The listing builds one solid part. Answer for the finished solid, in the listing's coordinates (mm). A direction names the side the tool comes from. Give positions to 0.01 mm unless a question says otherwise; leave off trailing zeros. Write each loop counter-clockwise with the first axis right and the second up, starting at its lowest first coordinate (ties: lowest second). Pieces come first, ordered by that corner, then holes. Notation, with made-up numbers: M 36,25 L 51,25 A26 ccw 51,40 Z; hole C -0.75,56 d4. An arc over 180 degrees is marked long. Return JSON: item names as keys, results as strings.
from build123d import *

# Parameters (mm, degrees)
F0_W = 99.274278
F0_H = 45.48195
F2_R = 20.32
F3_T = -2.54


with BuildPart() as f1:
    # F0 (on Right) → F1 (revolve)
    with BuildSketch(Plane.YZ):
        with Locations((49.637139, 22.740975)):
            Rectangle(F0_W, F0_H)
    revolve(axis=Axis((0, 49.637139, 0), (0, 1, 0)))

    # F2
    f2_edges = [f1.edges().sort_by_distance(p)[0] for p in [
        (0, 0, -45.48195),
    ]]
    fillet(f2_edges, radius=F2_R)

    # F3
    f3_openings = [f1.faces().sort_by_distance(p)[0] for p in [
        (0, 99.274278, 0),
    ]]
    offset(amount=F3_T, openings=f3_openings)


solid = f1.part
Item 1: A cutting plane is placed at C-C, the plane y = 79. Write down the section's boundary in (x, z), plus the area to 3 significant figures.
Geometry results:
{"outline": "C 0,0 d90.96; hole C 0,0 d85.88", "area": "706 mm2"}
Item 2: A cutting plane is placed at A-A, the plane z = 0. Write down the section's boundary in (x, y), plus the area to 3 significant figures.
Geometry results:
{"outline": "M -45.48,20.32 A20.32 ccw -25.16,0 L 25.16,0 A20.32 ccw 45.48,20.32 L 45.48,99.27 L 42.94,99.27 L 42.94,20.32 A17.78 cw 25.16,2.54 L -25.16,2.54 A17.78 cw -42.94,20.32 L -42.94,99.27 L -45.48,99.27 Z", "area": "681 mm2"}
Item 3: Find the intervals of material crossed by line 1 (X direction, y = 78.5, z = 0); line 2 (Y direction, x = -1, z = 25.5); line 3 (Z direction, x = -17, y = 66), in increasing order.
Geometry results:
{"line 1": "x = -45.48 to -42.94, 42.94 to 45.48", "line 2": "y = 0 to 2.54", "line 3": "z = -42.19 to -39.43, 39.43 to 42.19"}
Item 4: Given pin 1 Ø8 at (x, z) = (27, 19) entering from +Y; pin 2 Ø4 at (x, y) = (-27.5, 43.5) entering from -Z; pin 3 Ø4 at (y, z) = (21.5, -7) entering from -X, each flat-ended and moving along its own axis, determine where each tip first touches the part or whether it passes through.
Geometry results:
{"pin 1": "stops at y = 7.07", "pin 2": "stops at z = -37.66", "pin 3": "stops at x = -45.21"}
Item 5: Which of the six approach directions +Z, -Z, +X, -X, +Y, -Y give full straight-line access (tool end or side, diameter ignored) to faces 4 (the cylindrical face through (12.9, 60.35, 40.96)), 5 (the flat face through (0, 0, 0))?
Geometry results:
{"face 4": "+Y", "face 5": "+Z, -Z, +X, -X, -Y"}
Item 6: Determine the mould class of faces 1 (the flat face through (27.2, 99.274, -33.5)), 2 (the cylindrical face through (13.662, 60.35, 43.382)), 3 (the flat face through (0, 2.54, 0)) for opening direction Z: +Z half, -Z half, draft (parallel to the pull), parting line (faces both ways), or undercut.
Geometry results:
{"face 1": "draft", "face 2": "parting line", "face 3": "undercut"}
Item 7: A cutting plane is placed at B-B, the plane x = 0. Write down the section's boundary in (y, z), plus the area to 3 significant figures.
Geometry results:
{"outline": "M 0,-25.16 A20.32 ccw 20.32,-45.48 L 99.27,-45.48 L 99.27,-42.94 L 20.32,-42.94 A17.78 cw 2.54,-25.16 L 2.54,25.16 A17.78 cw 20.32,42.94 L 99.27,42.94 L 99.27,45.48 L 20.32,45.48 A20.32 ccw 0,25.16 Z", "area": "681 mm2"}
